For this review, use the dimensioned drawing (mm, ordinates from the lowest corner) and the shaded views. A direction names the side the tool comes from. Round coordinates to 2 decimals unless told otherwise and drop trailing zeros. Loops run counter-clockwise (first coordinate to the right, second up) from the corner with the lowest first, then second, coordinate; pieces in that order, holes last. Notation, with made-up numbers: (31.25, -21.5) -> (56.25, -21.5) arc R33 cw to (56.25, 11.5) -> close; hole circle Ø8 at (-6.75, 42). An arc over 180 degrees is marked (long way). Use one line per item in the form item = value. Start each with the question number.
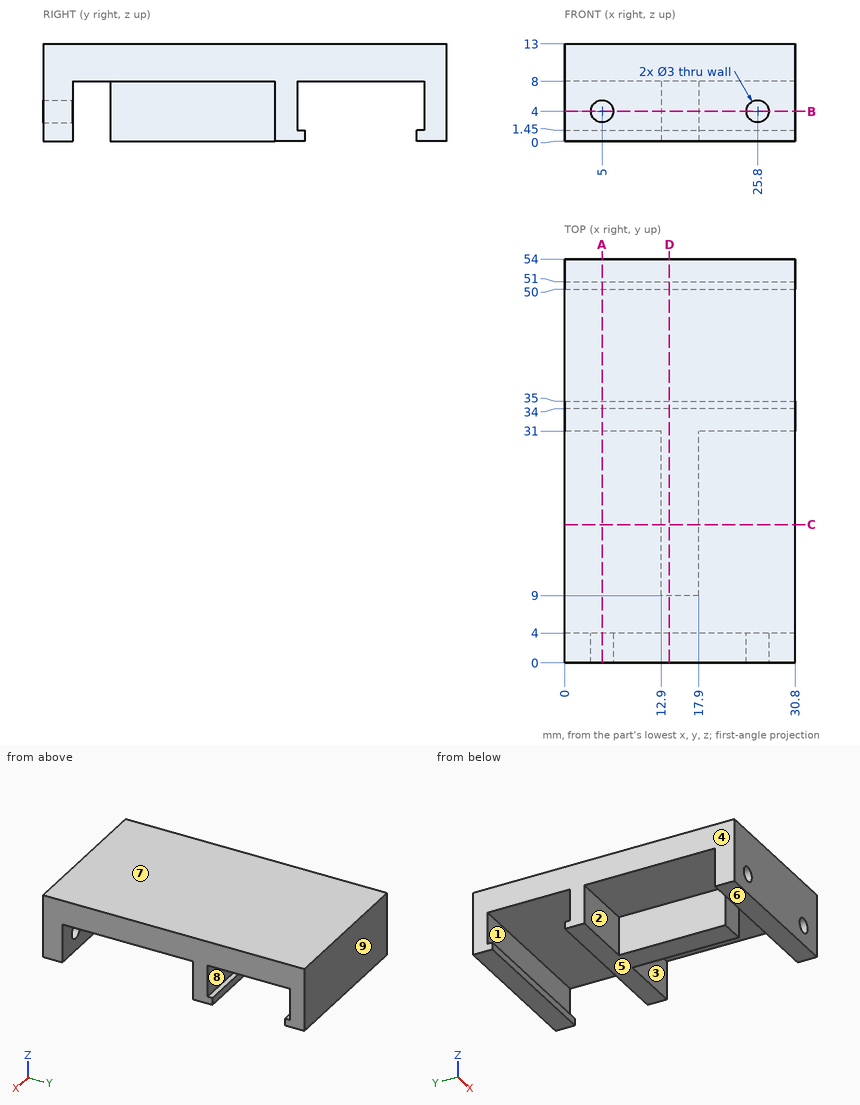
Item 1: Take a section at D-D on x = 14. Give the boundary of the cut face in (y, z).
Item 2: Machinability: for the marked faces 1, 2, 3, 4 and 5, which of the approach directions +Z, -Z, +X, -X, +Y, -Y give a long, thin tool a straight path to every point of the face, cutting with its end or side? Answer none if there is none.
Item 3: Take a section at C-C on y = 18.5. Give the boundary of the cut face in (x, z).
Item 4: Take a section at A-A on x = 5. Give the boundary of the cut face in (y, z), plus the area to 3 significant figures.
Item 5: Wall thickness on line 1 (Y direction, x = 15, z = 6.5); line 2 (X direction, y = 1.5, z = 4); line 3 (Y direction, x = 18, z = 1.75): over which ranges is each line inside the solid? List them lowest first.
Item 6: Draft analysis for pull direction Z (two halves, no side actions). For the marked faces 6, 7, 8 and 9, state which applies: +Z half, -Z half, draft (parallel to the pull), parting line (faces both ways), or undercut.
Item 7: Take a section at B-B on z = 4. Give the boundary of the cut face in (x, y), plus the area to 3 significant figures.
Item 8: For P1, Ø4, axis at y = 18, z = 2.5, coming from the +X side; P2, Ø2.5, axis at x = 5, z = 4, coming from the -Y side; P3, Ø5, axis at x = 7, y = 38, coming from the -Z side, all flat-tipped, find the tip position at first contact; note any pin that passes through.
Results:
q1.outline = (0, 0) -> (4, 0) -> (4, 8) -> (9, 8) -> (9, 0) -> (35, 0) -> (35, 1.45) -> (34, 1.45) -> (34, 8) -> (51, 8) -> (51, 1.45) -> (50, 1.45) -> (50, 0) -> (54, 0) -> (54, 13) -> (0, 13) -> close
q2.face_1 = +X, -X
q2.face_2 = -Z, -X
q2.face_3 = -Z, +X
q2.face_4 = +Z, -Z, -X, +Y, -Y
q2.face_5 = -Z, +X, -X, +Y, -Y
q3.outline = (0, 8) -> (12.9, 8) -> (12.9, 0) -> (17.9, 0) -> (17.9, 8) -> (30.8, 8) -> (30.8, 13) -> (0, 13) -> close
q4.outline = (0, 0) -> (4, 0) -> (4, 2.5) -> (0, 2.5) -> close; (0, 5.5) -> (4, 5.5) -> (4, 8) -> (31, 8) -> (31, 0) -> (35, 0) -> (35, 1.45) -> (34, 1.45) -> (34, 8) -> (51, 8) -> (51, 1.45) -> (50, 1.45) -> (50, 0) -> (54, 0) -> (54, 13) -> (0, 13) -> close
q4.area = 341 mm2
q5.line_1 = 0 to 4, 9 to 34, 51 to 54
q5.line_2 = 0 to 3.5, 6.5 to 24.3, 27.3 to 30.8
q5.line_3 = 0 to 4, 31 to 34, 51 to 54
q6.face_6 = -Z half
q6.face_7 = +Z half
q6.face_8 = undercut
q6.face_9 = draft
q7.outline = (0, 0) -> (3.5, 0) -> (3.5, 4) -> (0, 4) -> close; (0, 31) -> (12.9, 31) -> (12.9, 9) -> (17.9, 9) -> (17.9, 31) -> (30.8, 31) -> (30.8, 34) -> (0, 34) -> close; (0, 51) -> (30.8, 51) -> (30.8, 54) -> (0, 54) -> close; (6.5, 0) -> (24.3, 0) -> (24.3, 4) -> (6.5, 4) -> close; (27.3, 0) -> (30.8, 0) -> (30.8, 4) -> (27.3, 4) -> close
q7.area = 394 mm2
q8.P1 = 17.9
q8.P2 = 31
q8.P3 = 8
